from build123d import *

# Parameters (mm, degrees)
F1_DEPTH      = 5
F1_DEPTH_BACK = 5
F2_R          = 1
F3_DEPTH      = 32.001
F4_W          = 10
F4_H          = 50
F4_R          = 2
F5_DEPTH      = 10
F6_R          = 7.875
F7_DEPTH      = 10.001
F8_R          = 0.5


with BuildPart() as f1:
    # F0 (on Right) → F1 (new body, two sides)
    with BuildSketch(Plane.YZ) as f1_sk:
        with BuildLine():
            Line((15, 0.5), (15, 16))
            Line((15, 16), (-15, 16))
            Line((-15, 16), (-15, -16))
            Line((-15, -16), (15, -16))
            Line((15, -16), (15, -0.5))
            Line((15, -0.5), (7.859111, -0.5))
            ThreePointArc((7.859111, -0.5), (-7.875, 0), (7.859111, 0.5))
            Line((7.859111, 0.5), (15, 0.5))
        make_face()
    extrude(amount=F1_DEPTH)
    extrude(f1_sk.sketch, amount=-F1_DEPTH_BACK)

    # F2 (on face) → F3 (cut, through all)
    with BuildSketch(Plane.XY.offset(16)):
        with Locations((0, 11)):
            Circle(F2_R)
    extrude(amount=-F3_DEPTH, mode=Mode.SUBTRACT)

    # F4 (on face) → F5 (join)
    with BuildSketch(Plane(origin=(0, 0, -16), x_dir=(1, 0, 0), z_dir=(0, 0, -1))):
        Rectangle(F4_W, F4_H)
        with Locations((0, -20)):
            Circle(F4_R, mode=Mode.SUBTRACT)
        with Locations((0, 20)):
            Circle(F4_R, mode=Mode.SUBTRACT)
    extrude(amount=-F5_DEPTH)

    # F6 (on face) → F7 (cut, through all)
    with BuildSketch(Plane.YZ.offset(5)):
        Circle(F6_R)
    extrude(amount=-F7_DEPTH, mode=Mode.SUBTRACT)

    # F8
    f8_edges = [f1.edges().sort_by_distance(p)[0] for p in [
        (0, -15, 16),
        (0, 15, 16),
        (0, -25, -6),
        (0, 25, -6),
    ]]
    fillet(f8_edges, radius=F8_R)


solid = f1.part
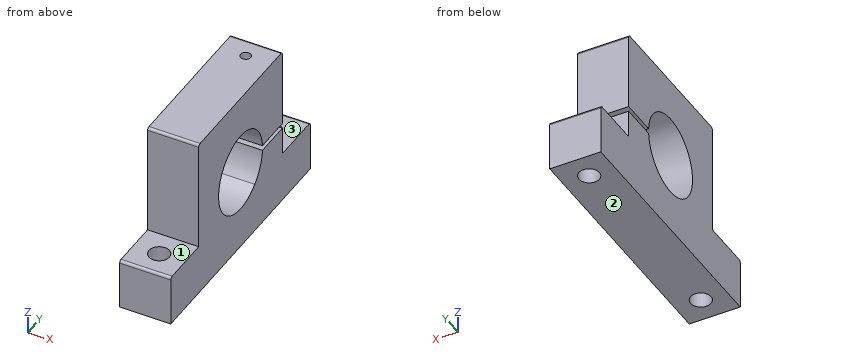
The model under review builds one solid part; all positions refer to its coordinate system, in mm. Face numbers are marked on the shaded views. A direction names the side the tool comes from. Give positions to 0.01 mm unless a question says otherwise; leave off trailing zeros. Write each loop counter-clockwise with the first axis right and the second up, starting at its lowest first coordinate (ties: lowest second). Pieces come first, ordered by that corner, then holes. Notation, with made-up numbers: M 72,14 L 80,14 A20 cw 80,37 Z; hole C 35,42 d5. An arc over 180 degrees is marked long. One line per question, with ' | ' between items. Start each with the question number.
Item 1: Wall thickness on line 1 (Y direction, x = 0, z = -13.75); line 2 (Y direction, x = 0, z = 1); line 3 (Y direction, x = 0, z = 10): over which ranges is each line inside the solid? List them lowest first. Write a range as from..to.
Item 2: We need section D-D on y = 11. Write out the cut boundary in (x, z).
Item 3: We need section A-A on z = -2. Write out the cut boundary in (x, y).
Item 4: We need section C-C on x = 0. Give the number of separate pieces and of enclosed holes in the cut face, plus the area to 3 significant figures.
Item 5: For the marked faces 1, 2 and 3, list the 3-axis set-ups (+Z, -Z, +X, -X, +Y, -Y) from which the entire face can be reached by the end or side of a thin tool; tool diameter is ignored.
Item 6: For pin 1 (3 mm diameter, centred on x = -1.5, z = -4, fed in from +Y); pin 2 (1.5 mm diameter, centred on x = -3, z = 6.5, fed in from -Y); pin 3 (3 mm diameter, centred on x = 2.5, y = -17.5, fed in from +Z), all flat-tipped, find the tip position at first contact; note any pin that passes through.
Item 7: We need section B-B on y = -20. Write out the cut boundary in (x, z), plus the area to 3 significant figures.
Results found:
1) line 1: y = -25..-22, -18..18, 22..25 | line 2: y = -15..-7.81, 7.81..10, 12..15 | line 3: y = -15..10, 12..15
2) outline: M -5,-16 L 5,-16 L 5,-0.5 L 1,-0.5 L 1,-6 L -1,-6 L -1,-0.5 L -5,-0.5 Z; M -5,0.5 L -1,0.5 L -1,16 L -5,16 Z; M 1,0.5 L 5,0.5 L 5,16 L 1,16 Z
3) outline: M -5,-15 L 5,-15 L 5,-7.62 L -5,-7.62 Z; M -5,7.62 L 5,7.62 L 5,15 L -5,15 Z; hole C 0,11 d2
4) separate pieces: 4 | enclosed holes: 0 | area: 836 mm2
5) face 1: +Z, +X, -X, -Y | face 2: -Z, +X, -X, +Y, -Y | face 3: +Z, +X, -X, +Y
6) pin 1: stops at y = 15 | pin 2: stops at y = -15 | pin 3: stops at z = -6
7) outline: M -5,-16 L -2,-16 L -2,-6 L -5,-6 Z; M 2,-16 L 5,-16 L 5,-6 L 2,-6 Z | area: 60.0 mm2
